Print and shaded views of the part. All mm, measured from the part's lowest x, y and z. A direction names the side the tool comes from. Coordinates: 2 decimals unless noted, no trailing zeros. Order: outer loops, then holes, each group sorted by start corner. A loop starts at its lowest first (then second) coordinate and runs counter-clockwise, first axis right, second up.
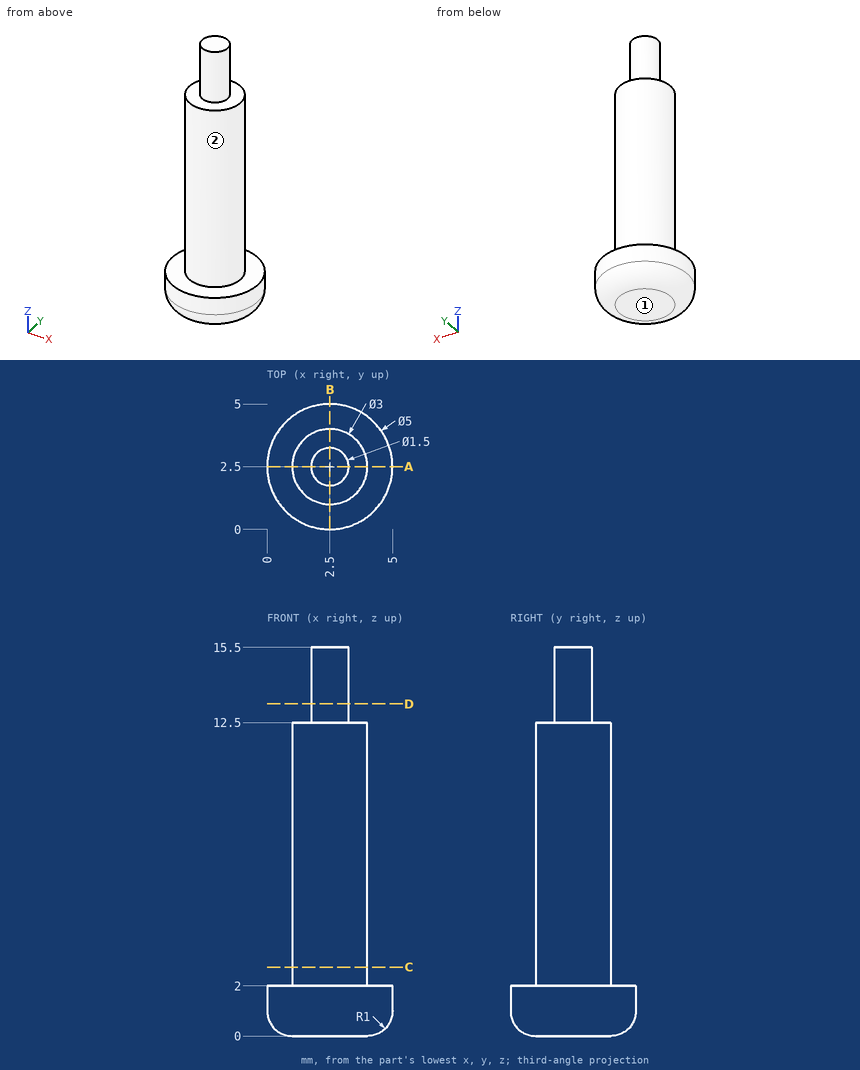
Q1. Cut at D-D, the plane z = 13.25. List the corners of the cut face in (x, y), plus the area to 3 significant figures.
Established:
outline: circle Ø1.5 at (2.5, 2.5)
area: 1.77 mm2
Q2. Cut at C-C, the plane z = 2.75. List the corners of the cut face in (x, y).
Established:
outline: circle Ø3 at (2.5, 2.5)
Q3. Cut at A-A, the plane y = 2.5. List the corners of the cut face in (x, z), plus the area to 3 significant figures.
Established:
outline: (0, 1) arc R1 ccw to (1, 0) - (4, 0) arc R1 ccw to (5, 1) - (5, 2) - (4, 2) - (4, 12.5) - (3.25, 12.5) - (3.25, 15.5) - (1.75, 15.5) - (1.75, 12.5) - (1, 12.5) - (1, 2) - (0, 2) - close
area: 45.6 mm2
Q4. Which spindle directions (+Z, -Z, +X, -X, +Y, -Y) get a long thin tool onto all of the face, cutting with end or side? Do the marked faces 1 and 2. Say none if no direction does.
Established:
face 1: -Z, +X, -X, +Y, -Y
face 2: +Z
Q5. Drop flat-ended pins along their axis: P1, Ø1, axis at y = 1, z = 11.5, coming from the -X side; P2, Ø1, axis at x = 2, z = 10.5, coming from the -Y side; P3, Ø2.5, axis at x = 2.5, y = 3.5, coming from the +Z side; P4, Ø1, axis at x = 2, z = 7.5, coming from the +Y side. Give the stop position or say it passes through.
Established:
P1: stops at x = 1.38
P2: stops at y = 1
P3: stops at z = 15.5
P4: stops at y = 4
Q6. Probe line 1 (X direction, y = 2.4, z = 11.25); line 2 (Z direction, x = 1, y = 2.05); line 3 (Z direction, x = 3.5, y = 1.9). List the from-to ranges inside material, lowest first.
Established:
line 1: x = 1 to 4
line 2: z = 0 to 2
line 3: z = 0 to 12.5
